Work out the finished part from the listing and answer in its coordinate system (mm). Face numbers are marked on the shaded views. A direction names the side the tool comes from. Round coordinates to 2 decimals unless told otherwise and drop trailing zeros. Write each loop counter-clockwise with the first axis right and the second up, starting at its lowest first coordinate (ties: lowest second). Pieces come first, ordered by that corner, then holes. Notation, with made-up numbers: M 82.25,-2.5 L 120.25,-2.5 A8 ccw 120.25,4.5 Z; hole C 8.5,3 d8. An arc over 180 degrees is marked long. Answer in a Markdown table with one row per item.
```python
from build123d import *

# Parameters (mm, degrees)
SKETCH1_R            = 1.5
BOSS_EXTRUDE1_DEPTH  = 10
FILLET1_R            = 1
M3_CLEARANCE_HOLE1_D = 3.2


with BuildPart() as part:
    # Sketch1 → Boss-Extrude1 (new body)
    with BuildSketch(Plane.XY):
        with BuildLine():
            Line((20.05, 5), (0, 5))
            ThreePointArc((0, 5), (-5, 0), (0, -5))
            Line((0, -5), (22, -5))
            Line((22, -5), (26.72989842, 1.621129525))
            Line((26.72989842, 1.621129525), (39.900164389, 7.036080522))
            Line((39.900164389, 7.036080522), (46.188488025, 4.540007042))
            Line((46.188488025, 4.540007042), (47.351030887, 4.342221563))
            Line((47.351030887, 4.342221563), (48.038244482, 5.300533868))
            Line((48.038244482, 5.300533868), (49.200787343, 5.102748388))
            Line((49.200787343, 5.102748388), (49.888000938, 6.061060693))
            Line((49.888000938, 6.061060693), (51.050543799, 5.863275214))
            Line((51.050543799, 5.863275214), (51.737757394, 6.821587519))
            Line((51.737757394, 6.821587519), (52.900300256, 6.623802039))
            Line((52.900300256, 6.623802039), (53.587513851, 7.582114344))
            Line((53.587513851, 7.582114344), (54.750056712, 7.384328864))
            Line((54.750056712, 7.384328864), (55.437270307, 8.34264117))
            Line((55.437270307, 8.34264117), (53.72608495, 12.504593197))
            Line((53.72608495, 12.504593197), (46.409029503, 15.837507263))
            Line((46.409029503, 15.837507263), (20.05, 5))
        make_face()
        Circle(SKETCH1_R, mode=Mode.SUBTRACT)
        with Locations((22, 0)):
            Circle(SKETCH1_R, mode=Mode.SUBTRACT)
    extrude(amount=BOSS_EXTRUDE1_DEPTH)

    # Fillet1
    fillet1_edges = [part.edges().sort_by_distance(p)[0] for p in [
        (22, -5, 5),
        (20.05, 5, 5),
        (46.409029503, 15.837507263, 5),
        (53.72608495, 12.504593197, 5),
        (55.437270307, 8.34264117, 5),
        (46.188488025, 4.540007042, 5),
        (39.900164389, 7.036080522, 5),
        (26.72989842, 1.621129525, 5),
    ]]
    fillet(fillet1_edges, radius=FILLET1_R)

    # M3 Clearance Hole1 (through all)
    with Locations(Plane.XY.offset(10)):
        with Locations((0, 0), (22, 0)):
            Hole(M3_CLEARANCE_HOLE1_D / 2)


solid = part.part
```
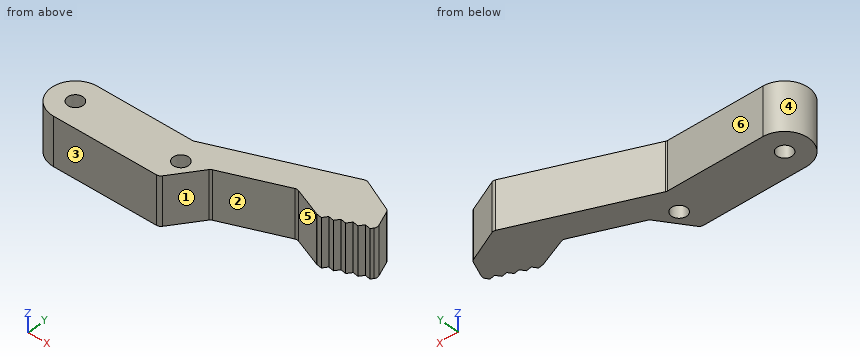
1. A tool of negligible diameter and unlimited length cuts with its end or side. For the marked faces 4, 5 and 6, from which of +Z, -Z, +X, -X, +Y, -Y can it reach the whole face along a straight path? Write none if from no direction.
Calculated:
| item | result |
|---|---|
| face 4 | +Z, -Z, -X |
| face 5 | +Z, -Z, -Y |
| face 6 | +Z, -Z, -X, +Y |
2. The part is cut by section A-A (z = 6.5). Count the separate pieces of the cut face and the enclosed holes in it, plus the area to 3 significant figures.
Calculated:
| item | result |
|---|---|
| separate pieces | 1 |
| enclosed holes | 2 |
| area | 488 mm² |
3. Given pin 1 (5 mm diameter, centred on y = 3, z = 3, fed in from -X); pin 2 (1 mm diameter, centred on y = 4.5, z = 2.5, fed in from +X); pin 3 (1.5 mm diameter, centred on x = 35.5, z = 6, fed in from -Y); pin 4 (1.9 mm diameter, centred on x = 0, y = 0, fed in from +Z), each flat-ended and moving along its own axis, determine where each tip first touches the part or whether it passes through.
Calculated:
| item | result |
|---|---|
| pin 1 | stops at x = -4.97 |
| pin 2 | stops at x = 47.82 |
| pin 3 | stops at y = 4.92 |
| pin 4 | passes through |
4. The part is cut by section D-D (y = -3). Determine the outline of the cut face in (x, z).
Calculated:
| item | result |
|---|---|
| outline | M -4,0 L 23.43,0 L 23.43,10 L -4,10 Z |
5. The part is cut by section B-B (y = 0). Determine the outline of the cut face in (x, z), plus the area to 3 significant figures.
Calculated:
| item | result |
|---|---|
| outline | M -5,0 L -1.6,0 L -1.6,10 L -5,10 Z; M 1.6,0 L 20.4,0 L 20.4,10 L 1.6,10 Z; M 23.6,0 L 25.57,0 L 25.57,10 L 23.6,10 Z |
| area | 242 mm² |
6. The part is cut by section C-C (x = 43). Determine the outline of the cut face in (y, z), plus the area to 3 significant figures.
Calculated:
| item | result |
|---|---|
| outline | M 5.81,0 L 14.44,0 L 14.44,10 L 5.81,10 Z |
| area | 86.3 mm² |
7. Consider line 1 along Y through (x, z) = (0, 6.75); line 2 along Y through (x, z) = (15.5, 1.75); line 3 along Y through (x, z) = (22, 9.25). Determine where each line is inside the solid, lowest interval first. Write a range as from..to.
Calculated:
| item | result |
|---|---|
| line 1 | y = -5..-1.6, 1.6..5 |
| line 2 | y = -5..5 |
| line 3 | y = -4.86..-1.6, 1.6..5.8 |
8. Determine the mould class of the marked faces 1, 2 and 3 for opening direction X: released by +X, released by -X, zero draft, split by the parting line, or undercut.
Calculated:
| item | result |
|---|---|
| face 1 | released by +X |
| face 2 | undercut |
| face 3 | zero draft |
